```python
from build123d import *

# Parameters (mm, degrees)
BOSS_EXTRUDE2_DEPTH = 3.175
FILLET1_R           = 1.27


# Read off the part's stored shape, not the designer's step: Boss-Extrude2
with BuildPart() as part:
    # Boss-Extrude2 outline → Boss-Extrude2 (new body)
    with BuildSketch(Plane.XY):
        with BuildLine():
            ThreePointArc((253.1745, 90.4748), (265.8745, 103.1748), (253.1745, 115.8748))
            Line((253.1745, 115.8748), (253.1745, 206.3496))
            Line((253.1745, 206.3496), (0, 206.3496))
            Line((0, 206.3496), (0, 0))
            Line((0, 0), (253.1745, 0))
            Line((253.1745, 0), (253.1745, 90.4748))
        make_face()
    extrude(amount=BOSS_EXTRUDE2_DEPTH)

    # Fillet1
    fillet1_edges = [part.edges().sort_by_distance(p)[0] for p in [
        (253.1745, 90.4748, 1.5875),
        (253.1745, 0, 1.5875),
        (0, 0, 1.5875),
        (0, 206.3496, 1.5875),
        (253.1745, 206.3496, 1.5875),
        (253.1745, 115.8748, 1.5875),
    ]]
    fillet(fillet1_edges, radius=FILLET1_R)


solid = part.part
```
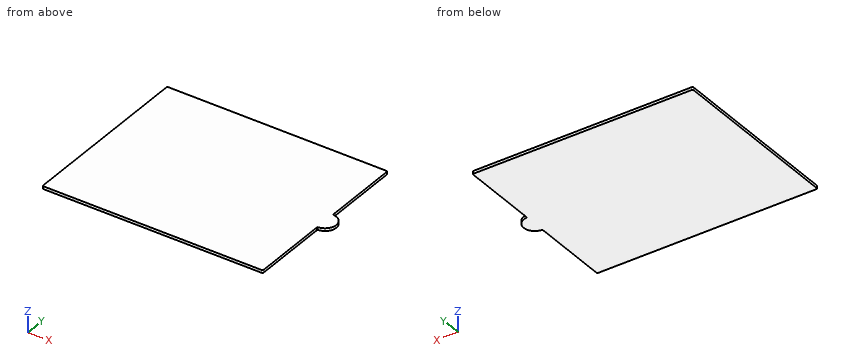
Source: CAD feature listing. Evaluate the final solid. Frame: model axes, mm. Give positions to 0.01 mm unless a question says otherwise; leave off trailing zeros. Loops run counter-clockwise (first coordinate to the right, second up) from the corner with the lowest first, then second, coordinate; pieces in that order, holes last. Notation, with made-up numbers: (-35.75, 17.25) -> (-9.75, 17.25) arc R25 ccw to (-9.75, 39.25) -> close; hole circle Ø6 at (15.25, -16.75). An arc over 180 degrees is marked (long way). Put each result on its own line as item: value. Start each with the question number.
1) Contact query for a flat-ended pin moving along its axis: P1, Ø1.6, axis at y = 176.5, z = 1.5, coming from the +X side. Output: stop coordinate, or through.
2) Cut plane A-A (z = 0.8). Return loops of the section in (x, y), then the cut area to 3 significant figures.
3) Cut plane B-B (y = 127). Return loops of the section in (x, z) (1 decimal), then the cut area to 3 significant figures.
4) Material intervals for probe 1 along X at (y, z) = (55, 1.2), sorted ascending.
5) Cut plane C-C (y = 93.5). Return loops of the section in (x, z) (3 decimals).
Results are:
1. P1: stops at x = 253.17
2. outline: (0, 1.27) arc R1.27 ccw to (1.27, 0) -> (251.9, 0) arc R1.27 ccw to (253.17, 1.27) -> (253.17, 89.26) arc R1.27 cw to (254.33, 90.53) arc R12.7 ccw to (254.33, 115.82) arc R1.27 cw to (253.17, 117.09) -> (253.17, 205.08) arc R1.27 ccw to (251.9, 206.35) -> (1.27, 206.35) arc R1.27 ccw to (0, 205.08) -> close
2. area: 52,500 mm2
3. outline: (0, 0) -> (253.2, 0) -> (253.2, 3.2) -> (0, 3.2) -> close
3. area: 804 mm2
4. probe 1: x = 0 to 253.17
5. outline: (0, 0) -> (261.402, 0) -> (261.402, 3.175) -> (0, 3.175) -> close
